Geometry: final body of the model. Coordinates: model frame, mm. A direction names the side the tool comes from. Give positions to 0.01 mm unless a question says otherwise; leave off trailing zeros. Loops run counter-clockwise (first coordinate to the right, second up) from the corner with the lowest first, then second, coordinate; pieces in that order, holes last. Notation, with made-up numbers: (79.5, -25.5) - (129.5, -25.5) arc R38 cw to (129.5, 13.5) - close; hole circle Ø1 at (33, 44). An arc over 180 degrees is marked (long way). Answer in a Markdown table with one row per item.
from build123d import *

# Parameters (mm, degrees)
CUT_EXTRUDE1_DEPTH = 3.5
SKETCH3_R          = 10
CUT_EXTRUDE2_DEPTH = 103.303470127
SKETCH4_W          = 6
SKETCH4_H          = 3.081008582
CUT_EXTRUDE3_DEPTH = 103.303470127


with BuildPart() as part:
    # Sketch1 → Revolve1 (revolve)
    with BuildSketch(Plane(origin=(0, 0, 0), x_dir=(1, 0, 0), z_dir=(0, 1, 0)), mode=Mode.PRIVATE) as revolve1_sk:
        Polygon((96, 0), (96, 19.5), (95.5, 20), (33, 20), (33, 25), (28, 25), (28, 20), (0.5, 20), (0, 19.5), (0, 0), align=None)
    revolve(revolve1_sk.sketch.rotate(Axis((0, 0, 0), (1, 0, 0)), 180), axis=Axis((0, 0, 0), (1, 0, 0)))

    # Sketch2 → Cut-Extrude1 (cut)
    with BuildSketch(Plane(origin=(0, 20, 0), x_dir=(1, 0, 0), z_dir=(0, 1, 0))):
        with BuildLine():
            Line((40, 6), (56, 6))
            ThreePointArc((56, 6), (62, 0), (56, -6))
            Line((56, -6), (40, -6))
            ThreePointArc((40, -6), (34, 0), (40, 6))
        make_face()
    extrude(amount=-CUT_EXTRUDE1_DEPTH, mode=Mode.SUBTRACT)

    # Sketch3 → Cut-Extrude2 (cut, through all)
    with BuildSketch(Plane.ZY):
        Circle(SKETCH3_R)
    extrude(amount=-CUT_EXTRUDE2_DEPTH, mode=Mode.SUBTRACT)

    # Sketch4 → Cut-Extrude3 (cut, through all)
    with BuildSketch(Plane.ZY):
        with Locations((0, -10.259495709)):
            Rectangle(SKETCH4_W, SKETCH4_H)
    extrude(amount=-CUT_EXTRUDE3_DEPTH, mode=Mode.SUBTRACT)


solid = part.part
Q1. First-contact query: pin 1 (8 mm diameter, centred on x = 81, y = -11.5, fed in from -Z); pin 2 (2 mm diameter, centred on x = 51, y = 17.5, fed in from -Z); pin 3 (3 mm diameter, centred on x = 51.5, y = 18, fed in from +Z). Flat tips, straight axial feed; report the tip coordinate or a pass-through.
Check values:
| item | result |
|---|---|
| pin 1 | z = -18.54 |
| pin 2 | z = -11.3 |
| pin 3 | z = 11.3 |
Q2. Cut plane B-B (y = 0). Output: boundary loops of the cut face in (x, z), and give its area (3 significant figures).
Check values:
| item | result |
|---|---|
| outline | (0, -19.5) - (0.5, -20) - (28, -20) - (28, -25) - (33, -25) - (33, -20) - (95.5, -20) - (96, -19.5) - (96, -10) - (0, -10) - close; (0, 10) - (96, 10) - (96, 19.5) - (95.5, 20) - (33, 20) - (33, 25) - (28, 25) - (28, 20) - (0.5, 20) - (0, 19.5) - close |
| area | 1,970 mm² |
Q3. Cut plane A-A (z = 0). Output: boundary loops of the cut face in (x, y), and give its area (3 significant figures).
Check values:
| item | result |
|---|---|
| outline | (0, -19.5) - (0.5, -20) - (28, -20) - (28, -25) - (33, -25) - (33, -20) - (95.5, -20) - (96, -19.5) - (96, -11.8) - (0, -11.8) - close; (0, 10) - (96, 10) - (96, 19.5) - (95.5, 20) - (62, 20) - (62, 16.5) - (34, 16.5) - (34, 20) - (33, 20) - (33, 25) - (28, 25) - (28, 20) - (0.5, 20) - (0, 19.5) - close |
| area | 1,700 mm² |
Q4. Material intervals for line 1 along Y through (x, z) = (23, 0); line 2 along Y through (x, z) = (57, 0); line 3 along Z through (x, y) = (7.5, -10), sorted ascending.
Check values:
| item | result |
|---|---|
| line 1 | -20 to -11.8, 10 to 20 |
| line 2 | -20 to -11.8, 10 to 16.5 |
| line 3 | -17.32 to -3, 3 to 17.32 |
Q5. Draft query along X for faces 1 (the cylindrical face through (14.06, -0.88, -19.98)), 2 (the cylindrical face through (62, 18, 0)), 3 (the flat face through (28, -17, -11)). Return one class per face: pulls with the +X half, pulls with the -X half, needs draft (parallel to the pull), parting line crosses it, or undercut.
Check values:
| item | result |
|---|---|
| face 1 | needs draft |
| face 2 | undercut |
| face 3 | pulls with the -X half |
Q6. Reachability of faces 4 (the flat face through (33, -17, 11)), 5 (the flat face through (96, -5, 9)), 6 (the flat face through (47, -11.8, 0)), 7 (the flat face through (48, 18, 6)), 8 (the flat face through (0, -5, -9)) from +Z, -Z, +X, -X, +Y, -Y: full face, straight path, thin tool, end or side. Return the list, or none.
Check values:
| item | result |
|---|---|
| face 4 | +X |
| face 5 | +Z, -Z, +X, +Y, -Y |
| face 6 | +X, -X |
| face 7 | +Y |
| face 8 | +Z, -Z, -X, +Y, -Y |
Q7. Cut plane C-C (x = 80). Output: boundary loops of the cut face in (y, z), and give its area (3 significant figures).
Check values:
| item | result |
|---|---|
| outline | circle Ø40 at (0, 0); hole (-11.8, -3) - (-9.54, -3) arc R10 ccw (long way) to (-9.54, 3) - (-11.8, 3) - close |
| area | 931 mm² |
